Job drawing, mm, ordinate dimensions from the low corner. One solid piece. A direction names the side the tool comes from. Give positions to 0.01 mm unless a question says otherwise; leave off trailing zeros. Loops run counter-clockwise (first coordinate to the right, second up) from the corner with the lowest first, then second, coordinate; pieces in that order, holes last.
Item 1: Which spindle directions (+Z, -Z, +X, -X, +Y, -Y) get a long thin tool onto all of the face, cutting with end or side? Do the marked faces 1, 2 and 3. Say none if no direction does.
Item 2: Saw through at A-A on z = 80.5. Give the cut face in (x, y).
Item 3: Probe probe 1 along X at (y, z) = (177, 10) (1 decimal); probe 2 along Y at (x, z) = (130.5, 71); probe 3 along Z at (x, y) = (11.5, 128.5). List the from-to ranges inside material, lowest first.
Item 4: Saw through at B-B on x = 40.5. Give the cut face in (y, z), plus the area to 3 significant figures.
Item 5: Saw through at C-C on y = 171.5. Give the cut face in (x, z).
Item 6: Saw through at D-D on x = 78. Give the cut face in (y, z).
Item 7: Mould opens along X. For the marked faces 4, 5, 6 and 7 say: released by +X, released by -X, zero draft, split by the parting line, or undercut.
Item 8: Drop a flat-ended pin along its axis: P1, Ø10, axis at x = 25, z = 60.5, coming from the -Y side. Give the stop position or say it passes through.
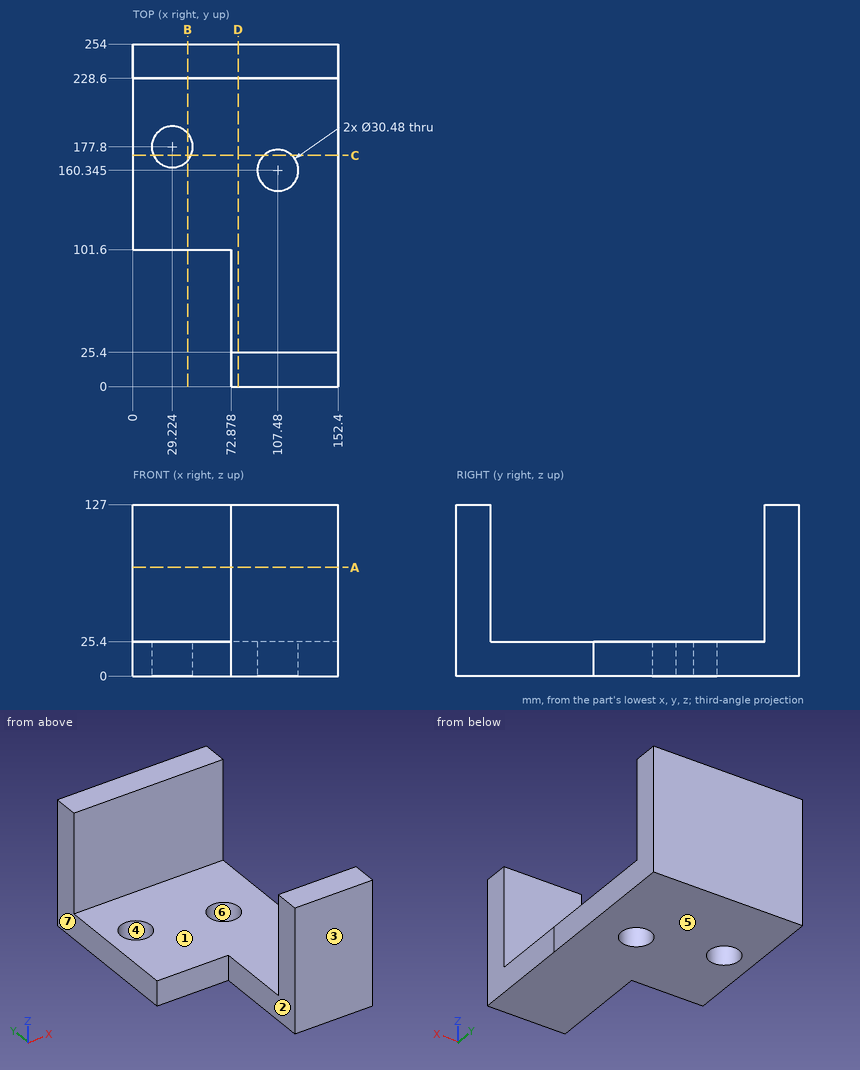
Results below:
1. face 1: +Z, +X, -X
1. face 2: +Z, -Z, -X, -Y
1. face 3: +Z, -Z, +X, -X, -Y
2. outline: (0, 228.6) - (152.4, 228.6) - (152.4, 254) - (0, 254) - close; (72.88, 0) - (152.4, 0) - (152.4, 25.4) - (72.88, 25.4) - close
3. probe 1: x = 0 to 14, 44.4 to 152.4
3. probe 2: y = 0 to 25.4, 228.6 to 254
3. probe 3: z = 0 to 25.4
4. outline: (101.6, 0) - (167.55, 0) - (167.55, 25.4) - (101.6, 25.4) - close; (188.05, 0) - (254, 0) - (254, 127) - (228.6, 127) - (228.6, 25.4) - (188.05, 25.4) - close
4. area: 5,930 mm2
5. outline: (0, 0) - (15.35, 0) - (15.35, 25.4) - (0, 25.4) - close; (43.1, 0) - (97.1, 0) - (97.1, 25.4) - (43.1, 25.4) - close; (117.86, 0) - (152.4, 0) - (152.4, 25.4) - (117.86, 25.4) - close
6. outline: (0, 0) - (254, 0) - (254, 127) - (228.6, 127) - (228.6, 25.4) - (25.4, 25.4) - (25.4, 127) - (0, 127) - close
7. face 4: undercut
7. face 5: zero draft
7. face 6: undercut
7. face 7: released by -X
8. P1: stops at y = 228.6
